Source: three-view drawing plus pictorial views. Frame: mm from the lowest corner of the part. A direction names the side the tool comes from. Round coordinates to 2 decimals unless told otherwise and drop trailing zeros. Order: outer loops, then holes, each group sorted by start corner. A loop starts at its lowest first (then second) coordinate and runs counter-clockwise, first axis right, second up. Notation, with made-up numbers: M 26,27 L 49,27 A15 ccw 49,32 Z; hole C 63.25,63.25 d7. An arc over 180 degrees is marked long. Return JSON: item names as keys, results as strings. Group by question number.
Q1. Mould query, pull axis X, two halves, no side actions, for the marked faces 1, 2 and 3. Classes: released by +X, released by -X, zero draft, split by the parting line, or undercut.
Q2. Cut plane C-C on y = 6. Output: boundary loops of the cut face in (x, z).
Q3. Ray query, probe 1 along X at (y, z) = (4.5, 4) (1 decimal); probe 2 along Y at (x, z) = (2.5, 1) (1 decimal); probe 3 along Y at (x, z) = (6.5, 6.5) (1 decimal). Return the intervals inside material, ascending.
Q4. Access query for the marked faces 4, 5 and 6. Directions: +Z, -Z, +X, -X, +Y, -Y. A direction counts if a zero-diameter tool reaches every point of the face in a straight line with its end or side. Return the directions, or none.
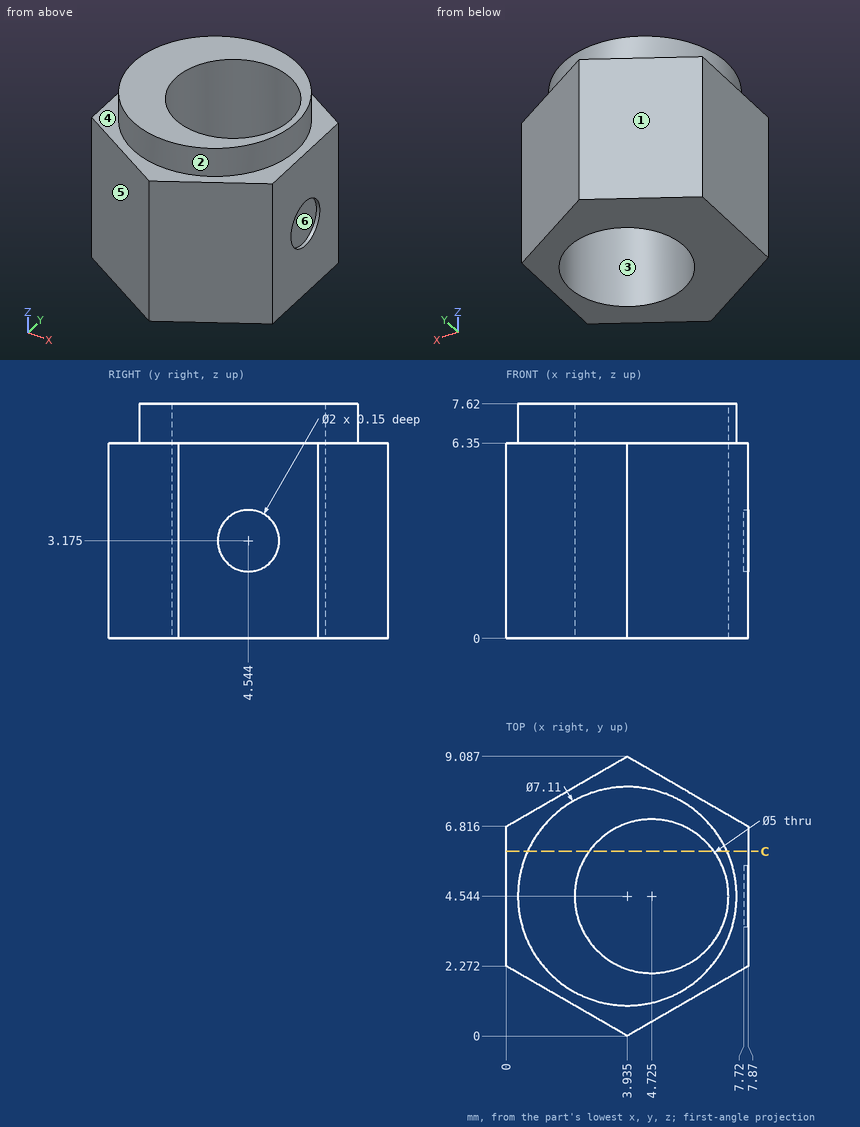
Result sheet:
{
 "1": {"face 1": "released by -X", "face 2": "split by the parting line", "face 3": "undercut"},
 "2": {"outline": "M 0,0 L 2.69,0 L 2.69,7.62 L 0.69,7.62 L 0.69,6.35 L 0,6.35 Z; M 6.76,0 L 7.87,0 L 7.87,6.35 L 7.18,6.35 L 7.18,7.62 L 6.76,7.62 Z"},
 "3": {"probe 1": "x = 0 to 2.2, 7.2 to 7.7", "probe 2": "y = 0.8 to 3.4, 5.7 to 8.3", "probe 3": "y = 2.1 to 2.8, 6.3 to 7"},
 "4": {"face 4": "+Z", "face 5": "+Z, -Z, -X, -Y", "face 6": "+X"}
}
